Autodesk Inventor part; units mm, degrees
ref_plane "YZ Plane" through (0, 0, 0) normal (1, 0, 0) x (0, 1, 0)
ref_plane "XZ Plane" through (0, 0, 0) normal (0, 1, 0) x (-1, 0, 0)
ref_plane "XY Plane" through (0, 0, 0) normal (0, 0, 1) x (1, 0, 0)
ref_plane "Work Plane2" through (-15, 5, -15) normal (-0.9487, 0, 0.3162) x (0, -1, 0)
sketch "Sketch3" plane through (-15, 5, -15) normal (-0.9487, 0, 0.3162) x (0, -1, 0)
  line L0 (0, 37.9473) -> (0, 0)
  line L1 (0, 0) -> (-5, 0)
  line L2 (-5, 0) -> (-5, 3)
  line L3 (-3, 5) -> (0, 5)
  line L4 (0, 0) -> (0, 5)
  arc A0 (-3, 5) -> (-5, 3) centre (-3, 3) ccw
  line L5 (0, 0) -> (5.0254, 0) construction
  line L6 (5, 0) -> (0, 0)
  line L7 (0, 0) -> (-5, -1.8199)
  line L8 (0, 0) -> (5.3209, 0) construction
  line L9 (-5, -1.8199) -> (-5, 0)
  line L10 (0, 0) -> (-3.2889, -1.1971)
  line L11 (0, 0) -> (-2.8191, -1.0261)
  line L12 (0, 0) -> (1.5391, -4.2286)
  line L13 (1.5391, -4.2286) -> (-2.6895, -5.7677)
  line L14 (-2.6895, -5.7677) -> (-2.8191, -1.0261)
  point P0 (5, 18.9737)
  point P1 (-5, 5)
  dimension "d5" = 5
  dimension "d6" = 5
  dimension "d7" = 2
  dimension "d9" = 160
  dimension "d12" = 3.5
  dimension "d20" = 3
  dimension "d21" = 4.5
extrude "Extrusion2" add sketch "Sketch3" against normal blind 30
ref_plane "Work Plane4" through (-16.8239, 7.6895, -20.4717) normal (0.1082, -0.9397, 0.3245) x (0.9487, 0, -0.3162)
sketch "Sketch5" plane through (-16.8239, 7.6895, -20.4717) normal (0.1082, -0.9397, 0.3245) x (0.9487, 0, -0.3162)
  line L0 (30, 4.5) -> (30, 0)
  line L1 (30, 0) -> (30, -0.5)
  line L2 (30, -0.5) -> (15, -0.5)
  line L3 (15, -0.5) -> (15, 2)
  circle A0 centre (15, 2) radius 1.5
  point P0 (9.4868, 20.6193)
  dimension "d24" = 0.5
  dimension "d25" = 15
  dimension "d26" = 2.5
  dimension "d27" = 3
extrude "Extrusion4" cut sketch "Sketch5" along normal blind 10
sketch "Sketch7" plane through (-15, 5, -15) normal (-0.9487, 0, 0.3162) x (0, -1, 0)
  line L0 (0, 0) -> (6.5506, 2.3842)
  line L1 (0, 0) -> (6.971, 0) construction
  line L2 (6.5506, 2.3842) -> (6.5506, -3.325)
  line L3 (6.5506, -3.325) -> (0, 0)
  point P0 (5, 18.9737)
  dimension "d34" = 20
extrude "Extrusion6" cut sketch "Sketch7" along normal blind 5 and the other way blind 40
fillet "Fillet2" radius 0.5 1 edges at (-2.5937, 7.6895, -25.2151)
sketch "Sketch8" plane through (-13.4189, 5, -10.2566) normal (0.3162, 0, 0.9487) x (0.9487, 0, -0.3162)
  line L0 (30, 0) -> (31.6228, 0)
  line L1 (30, 0) -> (36.1043, 0)
  line L2 (36.1043, 0) -> (36.1043, -10.0041)
  line L3 (36.1043, -10.0041) -> (30, -10.0041)
  line L4 (30, -10.0041) -> (30, 0)
  point P0 (9.4868, -5)
extrude "Extrusion7" cut sketch "Sketch8" along normal mid plane 20
ref_plane "Work Plane7" through (-15, 5, -15) normal (0.3162, 0, 0.9487) x (0.9487, 0, -0.3162)
sketch "Sketch10" plane through (-15, 5, -15) normal (0.3162, 0, 0.9487) x (0.9487, 0, -0.3162)
  line L0 (0, 0) -> (30, 0)
  line L1 (0, 0) -> (30, 0)
  line L2 (30, 0) -> (30, -5)
  line L3 (30, -5) -> (0, -5)
  line L4 (0, -5) -> (0, 0)
  line L5 (30, -5) -> (30, -10)
  line L6 (30, -10) -> (0, -5)
  point P0 (9.4868, -5)
  dimension "d49" = 30
  dimension "d50" = 5
  dimension "d51" = 5
extrude "Extrusion8" add sketch "Sketch10" along normal blind 5
sketch "Sketch11" plane through (15.0416, -5, -19.7434) normal (0.3162, 0, 0.9487) x (0.9487, 0, -0.3162)
  line L0 (-30, 10) -> (-30, 5)
  line L1 (-30, 5) -> (-30, 10)
  line L2 (-30, 10) -> (0, 5)
  line L3 (0, 0) -> (0, 10)
  line L4 (0, 0) -> (0, 5)
  line L5 (-30, 5) -> (0, 0)
  line L6 (0, 0) -> (-30, 5)
  point P0 (-20.5132, 5)
  dimension "d54" = 5
extrude "Extrusion9" add sketch "Sketch11" along normal blind 30
sketch "Sketch13" plane through (-13.4189, 5, -10.2566) normal (0.156, 0.9864, -0.052) x (0.9358, -0.1644, -0.3119)
  line L0 (30.4138, -30) -> (0, -30)
  line L1 (15.2069, -30) -> (15.2069, -15)
  circle A0 centre (15.2069, -15) radius 6.75
  line L2 (21.9569, -18.8971) -> (15.2069, -22.7942)
  line L3 (15.2069, -22.7942) -> (8.4569, -18.8971)
  line L4 (8.4569, -18.8971) -> (8.4569, -11.1029)
  line L5 (8.4569, -11.1029) -> (15.2069, -7.2058)
  line L6 (15.2069, -7.2058) -> (21.9569, -11.1029)
  line L7 (21.9569, -11.1029) -> (21.9569, -18.8971)
  circle A1 centre (15.2069, -15) radius 3.5
  point P0 (10.1797, -13.9737)
  point P1 (21.9569, -15)
  dimension "d58" = 13.5
  dimension "d57" = 15
  dimension "d59" = 7
extrude "Extrusion10" add sketch "Sketch13" along normal blind 4.25
properties part number "sem2_thumbmount2"
The model under review builds one solid part; all positions refer to its coordinate system, in mm. A direction names the side the tool comes from. Give positions to 0.01 mm unless a question says otherwise; leave off trailing zeros. Write each loop counter-clockwise with the first axis right and the second up, starting at its lowest first coordinate (ties: lowest second). Pieces come first, ordered by that corner, then holes. Notation, with made-up numbers: (26, 37) -> (50, 37) arc R12 cw to (50, 44) -> close; hole circle Ø7 at (44.5, 62). An arc over 180 degrees is marked (long way). Put each result on its own line as item: value.
(1) Tool access review of faces 1 (the flat face through (0.84, 5.13, -5.33)), 2 (the flat face through (-1.42, 8.89, -21.02)), 3 (the flat face through (7.138, 4.019, -7.488)): name each direction out of +Z, -Z, +X, -X, +Y, -Y from which nothing blocks a thin tool from reaching the whole face with its end or side.
Results are:
face 1: +Y
face 2: -Z, -X
face 3: +X
(2) To check wall thickness, follow probe 1 along Z at (x, y) = (2, 3.25); probe 2 along X at (y, z) = (5.25, -2); probe 3 along Z at (x, y) = (1.5, -0.5). State the ranges of each line that lie inside material, in increasing order. Write a range as from..to.
Results are:
probe 1: -20.67..-15.4, -6.86..16.23
probe 2: -1.59..2.63, 9.37..12.84
probe 3: -20.5..16.39
(3) The part is to be moulded in two halves that separate along X. For faces 4 (the flat face through (-14.7, 5.1, -14.1)), 5 (the flat face through (-1.182, 4.754, -20.317)), 6 (the flat face through (5.786, 6.954, 2.69)), say which applies: pulls with the +X half, pulls with the -X half, needs draft (parallel to the pull), parting line crosses it, or undercut.
Results are:
face 4: pulls with the -X half
face 5: undercut
face 6: pulls with the +X half
(4) We need section B-B, the plane x = 20.5. Give the boundary of the cut face in (y, z), and give its area (3 significant figures).
Results are:
outline: (-5, -3.37) -> (0, -3.37) -> (0.71, 10.06) -> (-4.29, 10.06) -> close
area: 67.1 mm²
(5) For pin 1 Ø4 at (x, y) = (8, 2.5) entering from -Z; pin 2 Ø10 at (x, z) = (-2.5, -15.5) entering from -Y; pin 3 Ø1 at (x, y) = (10.5, 0) entering from +Z, all flat-tipped, find the tip position at first contact; note any pin that passes through.
Results are:
pin 1: z = -27.77
pin 2: y = -2.84
pin 3: z = 13.56
(6) We need section C-C, the plane z = 8. Give the boundary of the cut face in (x, y), and give its area (3 significant figures).
Results are:
outline: (-7.33, 0) -> (24.29, -5) -> (24.29, 0) -> (-7.33, 5) -> close
area: 158 mm²
